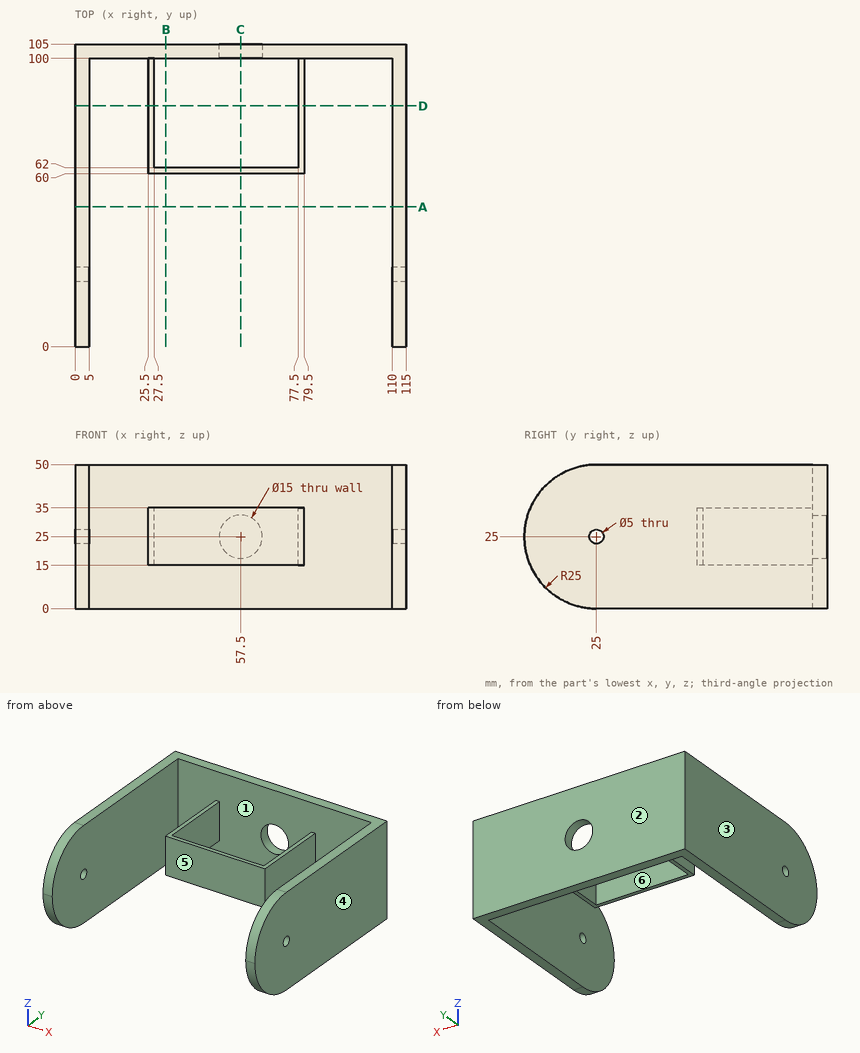
Verification items for this drawing (mm, ordinates from the low corner). A direction names the side the tool comes from. Give positions to 0.01 mm unless a question says otherwise; leave off trailing zeros. Write each loop counter-clockwise with the first axis right and the second up, starting at its lowest first coordinate (ties: lowest second). Pieces come first, ordered by that corner, then holes. Notation, with made-up numbers: (75, 77) - (85, 77) arc R11 ccw to (85, 98) - close; hole circle Ø7 at (56, 52). An arc over 180 degrees is marked (long way). Answer as a JSON object with one key per item and string values. Group by question number.
1) Sectioned sample at B-B (x = 31.5). Record the cut outline in (y, z).
2) Sectioned sample at A-A (y = 48.5). Record the cut outline in (x, z).
3) Sectioned sample at C-C (x = 57.5). Record the cut outline in (y, z), then the cut area to 3 significant figures.
4) Depth check by flat-ended pin: P1, Ø4, axis at y = 25, z = 25, coming from the -X side; P2, Ø8, axis at x = 43.5, z = 41, coming from the -Y side; P3, Ø25, axis at x = 67.5, z = 13, coming from the -Y side; P4, Ø1.5, axis at x = 55, z = 21.5, coming from the +Y side. Enter the tip coordinate at first touch or a pass-through.
5) Release check for a two-part mould opening along X. For the marked faces 1, 2 and 3 record: pulls with the +X half, pulls with the -X half, needs draft (parallel to the pull), parting line crosses it, or undercut.
6) Sectioned sample at D-D (y = 83.5). Record the cut outline in (x, z), then the cut area to 3 significant figures.
7) Access from +Z, -Z, +X, -X, +Y, -Y to the whole of each face (thin tool, end or side, straight path). Record for the marked faces 4, 5 and 6.
8) Thickness scan on probe 1 along X at (y, z) = (59, 11.5); probe 2 along Y at (x, z) = (49, 20.5); probe 3 along Z at (x, y) = (57.5, 103.6). Record the ranges inside material, lowest first. Write a range as from..to.
Geometry results:
{
 "1": {"outline": "(60, 15) - (62, 15) - (62, 35) - (60, 35) - close; (100, 0) - (105, 0) - (105, 50) - (100, 50) - close"},
 "2": {"outline": "(0, 0) - (5, 0) - (5, 50) - (0, 50) - close; (110, 0) - (115, 0) - (115, 50) - (110, 50) - close"},
 "3": {"outline": "(60, 15) - (62, 15) - (62, 35) - (60, 35) - close; (100, 0) - (105, 0) - (105, 17.5) - (100, 17.5) - close; (100, 32.5) - (105, 32.5) - (105, 50) - (100, 50) - close", "area": "215 mm^2"},
 "4": {"P1": "passes through", "P2": "stops at y = 100", "P3": "stops at y = 60", "P4": "stops at y = 62"},
 "5": {"face 1": "undercut", "face 2": "needs draft", "face 3": "pulls with the -X half"},
 "6": {"outline": "(0, 0) - (5, 0) - (5, 50) - (0, 50) - close; (25.5, 15) - (27.5, 15) - (27.5, 35) - (25.5, 35) - close; (77.5, 15) - (79.5, 15) - (79.5, 35) - (77.5, 35) - close; (110, 0) - (115, 0) - (115, 50) - (110, 50) - close", "area": "580 mm^2"},
 "7": {"face 4": "+Z, -Z, +X, +Y, -Y", "face 5": "+Z, -Z, -Y", "face 6": "+Z, -Z"},
 "8": {"probe 1": "x = 0..5, 110..115", "probe 2": "y = 60..62, 100..105", "probe 3": "z = 0..17.5, 32.5..50"}
}
